Could you check a few things on this model? Use its own coordinates, in mm. A direction names the side the tool comes from. Give positions to 0.01 mm unless a question says otherwise; leave off trailing zeros. Loops run counter-clockwise (first coordinate to the right, second up) from the corner with the lowest first, then second, coordinate; pieces in that order, holes last. Notation, with made-up numbers: (36, 87.25) - (67, 87.25) arc R22 ccw to (67, 98.25) - close; hole circle Ø10 at (-37.75, 13.5). An arc over 180 degrees is marked (long way). One line per item, written item: value. Start each with the question number.
Q1. If we mould it in two halves opening along Y, with no side actions, what happens to faces 4 (the face through (-3, -15, 0)), 5 (the face through (139.043, -36.931, 2.028)), 6 (the face through (135, -46.31, 2.03))? For each: released by +Y, released by -Y, zero draft, split by the parting line, or undercut.
Q2. If I drill on line 1 (Y direction, x = -48, z = 0.6); line 2 (Y direction, x = -106, z = 1.6); line 3 (X direction, y = -5, z = 1.75), over which ranges is the centre line in solid material (lowest first)? Write a range as from..to.
Q3. For faces 1 (the face through (21.655, 0.117, 2.028)), 2 (the face through (-135, -46.31, 2.03)), 3 (the face through (-3, -15, 4)), which set-ups out of +Z, -Z, +X, -X, +Y, -Y let a thin tool reach every point of the face, with its end or its side?
Q4. I'm going to push flat-ended pins straight in: P1, Ø3.5, axis at x = 192, y = -62, coming from the +Z side; P2, Ø1.2, axis at y = 3.5, z = 2.5, coming from the +X side; P3, Ø1.2, axis at y = 4, z = 1, coming from the -X side; P4, Ø2, axis at x = -185.5, z = 2, coming from the +Y side. Where does each tip first touch, or does it pass through?
Q5. I want a section at B-B (z = 2.8). Count the separate pieces of the cut face and the enclosed holes in it, then the cut area to 3 significant figures.
Q6. I want a section at A-A (y = 4). Please give me the cut outline in (x, z).
```python
from build123d import *

# Parameters (mm, degrees)
SKETCH_1_W          = 232
SKETCH_1_H          = 40
SKETCH_1_R          = 2.1
EXTRUDE_1_DEPTH     = 4
SKETCH_2_R          = 3.1
EXTRUDE_2_DEPTH     = 4
SKETCH_4_R          = 2.1
CUT_EXTRUDE_2_DEPTH = 10
FILLET_1_R          = 3
FILLET_2_R          = 10
SKETCH_6_R          = 2.05
SKETCH_6_R_2        = 3.1
CUT_EXTRUDE_4_DEPTH = 209.844439715
CUT_EXTRUDE_5_DEPTH = 10
FILLET_3_R          = 1


with BuildPart() as part:
    # 草图1 → 凸台-拉伸1 (new body)
    with BuildSketch(Plane.XY):
        Rectangle(SKETCH_1_W, SKETCH_1_H)
        with Locations((-47.5, 12.5)):
            Circle(SKETCH_1_R, mode=Mode.SUBTRACT)
        with Locations((47.5, 12.5)):
            Circle(SKETCH_1_R, mode=Mode.SUBTRACT)
        with Locations((-47.5, -12.5)):
            Circle(SKETCH_1_R, mode=Mode.SUBTRACT)
        with Locations((47.5, -12.5)):
            Circle(SKETCH_1_R, mode=Mode.SUBTRACT)
    extrude(amount=EXTRUDE_1_DEPTH)

    # 草图2 → 凸台-拉伸2 (add)
    # profile 1 of 2: a face of its own
    with BuildSketch(Plane.XY.offset(4)):
        Polygon((-116, 20), (-168, -52), (-196, -52), (-196, -72), (-153.555555556, -72), (-116, -20), align=None)
        with Locations((-142, -36)):
            Circle(SKETCH_2_R, mode=Mode.SUBTRACT)
    # profile 2 of 2: a face of its own
    with BuildSketch(Plane.XY.offset(4)):
        Polygon((116, 20), (168, -52), (196, -52), (196, -72), (153.555555556, -72), (116, -20), align=None)
        with Locations(Location((142, -36, 0), (0, 0, 180))):
            Circle(SKETCH_2_R, mode=Mode.SUBTRACT)
    extrude(amount=-EXTRUDE_2_DEPTH)

    # 草图4 → 切除-拉伸2 (cut)
    with BuildSketch(Plane.XY.offset(4)):
        with Locations((-106, 12.5)):
            Circle(SKETCH_4_R)
        with Locations((-106, -12.5)):
            Circle(SKETCH_4_R)
        with Locations((106, 12.5)):
            Circle(SKETCH_4_R)
        with Locations((106, -12.5)):
            Circle(SKETCH_4_R)
    extrude(amount=-CUT_EXTRUDE_2_DEPTH, mode=Mode.SUBTRACT)

    # 圆角1
    fillet_1_edges = [part.edges().sort_by_distance(p)[0] for p in [
        (-196, -72, 2),
        (-196, -52, 2),
        (196, -52, 2),
        (196, -72, 2),
    ]]
    fillet(fillet_1_edges, radius=FILLET_1_R)

    # 圆角2
    fillet_2_edges = [part.edges().sort_by_distance(p)[0] for p in [
        (-153.555555556, -72, 2),
        (-168, -52, 2),
        (168, -52, 2),
        (153.555555556, -72, 2),
        (116, -20, 2),
        (-116, -20, 2),
        (-116, 20, 2),
        (116, 20, 2),
    ]]
    fillet(fillet_2_edges, radius=FILLET_2_R)

    # 草图6 → 切除-拉伸4 (cut, through all)
    with BuildSketch(Plane.XY.offset(4)):
        with Locations((-192, -62)):
            Circle(SKETCH_6_R)
        with Locations((-172, -62)):
            Circle(SKETCH_6_R)
        with Locations(Location((172, -62, 0), (0, 0, 180))):
            Circle(SKETCH_6_R)
        with Locations(Location((192, -62, 0), (0, 0, 180))):
            Circle(SKETCH_6_R)
        with Locations((-182, -62)):
            Circle(SKETCH_6_R_2)
        with Locations((182, -62)):
            Circle(SKETCH_6_R_2)
    extrude(amount=-CUT_EXTRUDE_4_DEPTH, mode=Mode.SUBTRACT)

    # 草图5 → 切除-拉伸5 (cut)
    with BuildSketch(Plane.XY.offset(4)):
        Polygon((-40, 14), (-40, -14), (-3, -14), align=None)
        Polygon((-30.057050493, 14), (-3, -6.475605779), (-3, 14), align=None)
        Polygon((40, -14), (3, -14), (40, 14), align=None)
        Polygon((3, -6.475605779), (3, 14), (30.057050493, 14), align=None)
    extrude(amount=-CUT_EXTRUDE_5_DEPTH, mode=Mode.SUBTRACT)

    # 圆角3
    fillet_3_edges = [part.edges().sort_by_distance(p)[0] for p in [
        (-3, 14, 2),
        (-3, -6.475605779, 2),
        (-30.057050493, 14, 2),
        (3, 14, 2),
        (30.057050493, 14, 2),
        (3, -6.475605779, 2),
        (3, -14, 2),
        (40, 14, 2),
        (40, -14, 2),
        (-3, -14, 2),
        (-40, -14, 2),
        (-40, 14, 2),
    ]]
    fillet(fillet_3_edges, radius=FILLET_3_R)


solid = part.part
```
Worked answers:
1. face 4: zero draft
1. face 5: undercut
1. face 6: released by -Y
2. line 1: y = -20..-14.54, -10.46..10.46, 14.54..20
2. line 2: y = -20..-14.6, -10.4..10.4, 14.6..20
2. line 3: x = -134.06..-40, -14.89..-4.95, -3.16..3.16, 4.95..14.89, 40..134.06
3. face 1: +Z, -Z
3. face 2: +Z, -Z, -Y
3. face 3: +Z, +X, -X, +Y, -Y
4. P1: passes through
4. P2: stops at x = 128.35
4. P3: stops at x = -127.99
4. P4: stops at y = -52
5. separate pieces: 1
5. enclosed holes: 20
5. area: 12,400 mm²
6. outline: (-127.56, 0) - (-40, 0) - (-40, 4) - (-127.56, 4) - close; (-26.79, 0) - (-16.84, 0) - (-16.84, 4) - (-26.79, 4) - close; (-3, 0) - (3, 0) - (3, 4) - (-3, 4) - close; (16.84, 0) - (26.79, 0) - (26.79, 4) - (16.84, 4) - close; (40, 0) - (127.56, 0) - (127.56, 4) - (40, 4) - close
